Check sheet for the modelled part. Datum: model origin and axes. Units: mm. A direction names the side the tool comes from. Coordinates: 2 decimals unless noted, no trailing zeros. Order: outer loops, then holes, each group sorted by start corner. A loop starts at its lowest first (then second) coordinate and runs counter-clockwise, first axis right, second up.
from build123d import *

# Parameters (mm, degrees)
F1_DEPTH = 12.7
F3_DEPTH = 12.701
F5_DEPTH = 12.701


with BuildPart() as f1:
    # F0 (on Right) → F1 (new body)
    with BuildSketch(Plane.YZ):
        Polygon((12.7, 25.4), (-177.8, 25.4), (-177.8, 0), (146.05, 0), (177.8, 0), (177.8, 25.4), align=None)
        with BuildLine():
            Line((38.1, 50.8), (12.7, 25.4))
            Line((12.7, 25.4), (177.8, 25.4))
            Line((177.8, 25.4), (177.8, 228.6))
            Line((177.8, 228.6), (146.05, 228.6))
            Line((146.05, 228.6), (146.05, 57.15))
            ThreePointArc((146.05, 57.15), (144.190128, 52.659872), (139.7, 50.8))
            Line((139.7, 50.8), (38.1, 50.8))
        make_face()
    extrude(amount=F1_DEPTH)

    # F2 (on face) → F3 (cut, through all)
    with BuildSketch(Plane.YZ.offset(12.7)):
        with BuildLine():
            ThreePointArc((166.1414, 209.55), (161.925, 213.7664), (157.7086, 209.55))
            Line((157.7086, 209.55), (157.7086, 114.3))
            ThreePointArc((157.7086, 114.3), (161.925, 110.0836), (166.1414, 114.3))
            Line((166.1414, 114.3), (166.1414, 209.55))
        make_face()
    extrude(amount=-F3_DEPTH, mode=Mode.SUBTRACT)

    # F4 (on face) → F5 (cut, through all)
    with BuildSketch(Plane.YZ.offset(12.7)):
        with BuildLine():
            Line((152.4, 38.1), (50.8, 38.1))
            ThreePointArc((50.8, 38.1), (44.45, 31.75), (50.8, 25.4))
            Line((50.8, 25.4), (152.4, 25.4))
            ThreePointArc((152.4, 25.4), (158.75, 31.75), (152.4, 38.1))
        make_face()
    extrude(amount=-F5_DEPTH, mode=Mode.SUBTRACT)


solid = f1.part
(1) Release check for a two-part mould opening along Y. For faces 1 (the flat face through (6, 177.8, 113)), 2 (the cylindrical face through (6.26, 144.24, 52.71)), 3 (the cylindrical face through (6.439, 161.832, 110.085)), 4 (the flat face through (12.7, 65, 47)) record: +Y half, -Y half, draft (parallel to the pull), parting line (faces both ways), or undercut.
Filled in:
face 1: +Y half
face 2: -Y half
face 3: undercut
face 4: draft
(2) Thickness scan on probe 1 along Z at (x, y) = (5.25, 118.5); probe 2 along Y at (x, z) = (10.5, 193); probe 3 along Z at (x, y) = (2, 12). Record the ranges inside material, lowest first.
Filled in:
probe 1: z = 0 to 25.4, 38.1 to 50.8
probe 2: y = 146.05 to 157.71, 166.14 to 177.8
probe 3: z = 0 to 25.4
(3) Cross-section at B-B (y = 97.5). Enter the section's corners in (x, z), and give its area (3 significant figures).
Filled in:
outline: (0, 0) - (12.7, 0) - (12.7, 25.4) - (0, 25.4) - close; (0, 38.1) - (12.7, 38.1) - (12.7, 50.8) - (0, 50.8) - close
area: 484 mm2
(4) Go/stop test with flat-tipped pins: P1, Ø4, axis at x = 6, z = 155, coming from the -Y side; P2, Ø6.5, axis at x = 3.5, y = -95.5, coming from the +Z side; P3, Ø4, axis at x = 6, y = -97.5, coming from the -Z side; P4, Ø3, axis at x = 8.5, y = 125, coming from the +Z side. Record where each tip stops, or that it passes through.
Filled in:
P1: stops at y = 146.05
P2: stops at z = 25.4
P3: stops at z = 0
P4: stops at z = 50.8
(5) Cross-section at C-C (x = 4). Enter the section's corners in (y, z) (3 decimals).
Filled in:
outline: (-177.8, 0) - (177.8, 0) - (177.8, 228.6) - (146.05, 228.6) - (146.05, 57.15) arc R6.35 cw to (139.7, 50.8) - (38.1, 50.8) - (12.7, 25.4) - (-177.8, 25.4) - close; hole (50.8, 25.4) - (152.4, 25.4) arc R6.35 ccw to (152.4, 38.1) - (50.8, 38.1) arc R6.35 ccw to start; hole (157.709, 114.3) arc R4.216 ccw to (166.141, 114.3) - (166.141, 209.55) arc R4.216 ccw to (157.709, 209.55) - close
(6) Tool access check on faces 5 (the cylindrical face through (6.44, 158.75, 31.61)), 6 (the flat face through (6, 146.05, 144)), 7 (the flat face through (6, 162, 228.6)). Record the directions out of +Z, -Z, +X, -X, +Y, -Y that give a thin tool (end or side, any length) a straight path to the whole face; none if there is none.
Filled in:
face 5: +X, -X
face 6: +Z, +X, -X, -Y
face 7: +Z, +X, -X, +Y, -Y
(7) Cross-section at A-A (z = 31.75). Enter the section's corners in (x, y).
Filled in:
outline: (0, 19.05) - (12.7, 19.05) - (12.7, 44.45) - (0, 44.45) - close; (0, 158.75) - (12.7, 158.75) - (12.7, 177.8) - (0, 177.8) - close
